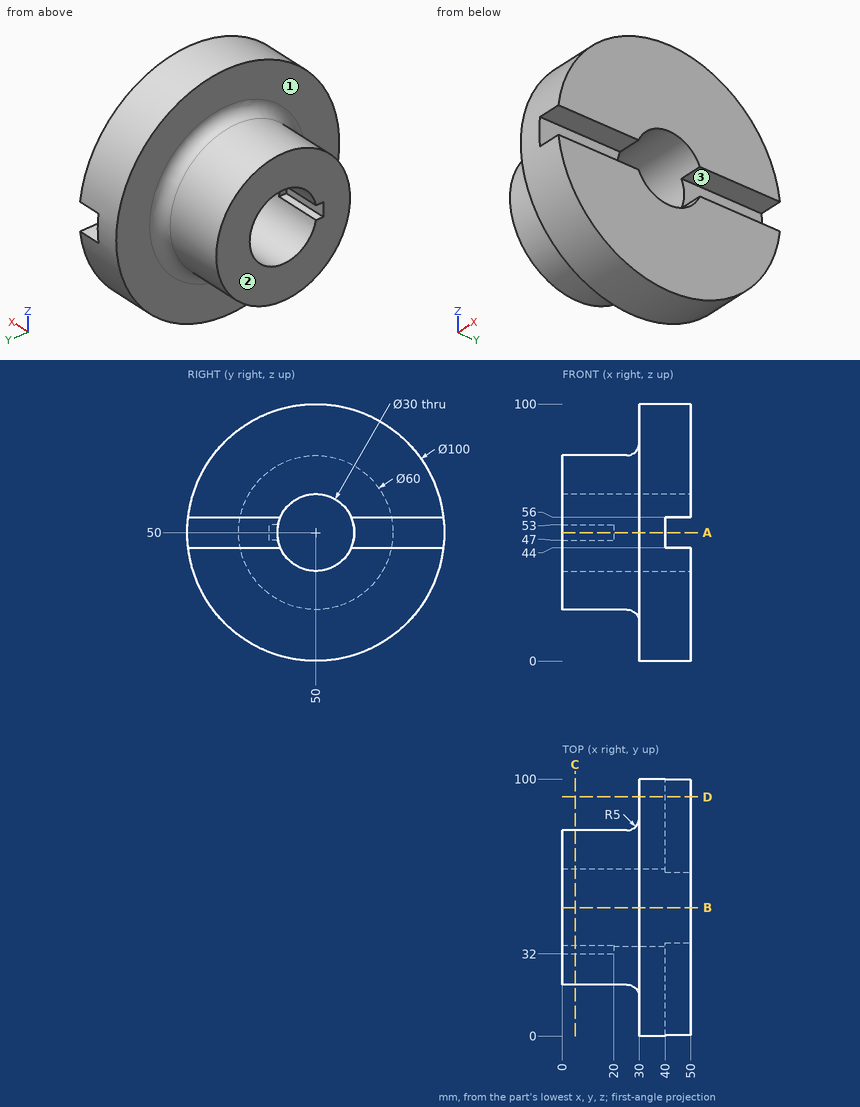
Geometry: see drawing. Coordinates: mm, zero at the bounding-box minimum. A direction names the side the tool comes from. Round coordinates to 2 decimals unless told otherwise and drop trailing zeros. Loops run counter-clockwise (first coordinate to the right, second up) from the corner with the lowest first, then second, coordinate; pieces in that order, holes last. Notation, with made-up numbers: (20.25, -20.5) -> (29.25, -20.5) arc R30 cw to (29.25, 14.5) -> close; hole circle Ø4 at (37.25, 10.25). An arc over 180 degrees is marked (long way). Write each question's results on one line, items separated by ' | '.
1. First-contact query: P1, Ø1.7, axis at y = 34, z = 49, coming from the -X side; P2, Ø3, axis at x = 39.5, z = 39, coming from the -Y side; P3, Ø11, axis at x = 44.5, y = 25, coming from the -Z side. Flat tips, straight axial feed; report the tip coordinate or a pass-through.
Geometry results:
P1: x = 20 | P2: y = 0.91 | P3: z = 3.96
2. Set-up query: the marked faces 1, 2 and 3. Return all of +Z, -Z, +X, -X, +Y, -Y with unobstructed straight access to the full face (end or side cutting, diameter ignored); none if empty.
Geometry results:
face 1: -X | face 2: +Z, -Z, -X, +Y, -Y | face 3: +X, +Y, -Y
3. Section A-A (z = 50). Return loops of the section in (x, y), and give its area (3 significant figures).
Geometry results:
outline: (0, 20) -> (25, 20) arc R5 cw to (30, 15) -> (30, 0) -> (40, 0) -> (40, 35) -> (20, 35) -> (20, 32) -> (0, 32) -> close; (0, 65) -> (40, 65) -> (40, 100) -> (30, 100) -> (30, 85) arc R5 cw to (25, 80) -> (0, 80) -> close | area: 1,550 mm2
4. Section C-C (x = 5). Return loops of the section in (y, z), and give its area (3 significant figures).
Geometry results:
outline: circle Ø60 at (50, 50); hole (32, 47) -> (35.3, 47) arc R15 ccw (long way) to (35.3, 53) -> (32, 53) -> close | area: 2,100 mm2
5. Ray query, line 1 (Z direction, x = 39, y = 50); line 2 (Z direction, x = 10, y = 50); line 3 (X direction, y = 45, z = 95). Return the intervals inside material, ascending. Write a range as from..to.
Geometry results:
line 1: 0..35, 65..100 | line 2: 20..35, 65..80 | line 3: 30..50
6. Section B-B (y = 50). Return loops of the section in (x, z).
Geometry results:
outline: (0, 20) -> (25, 20) arc R5 cw to (30, 15) -> (30, 0) -> (50, 0) -> (50, 35) -> (0, 35) -> close; (0, 65) -> (50, 65) -> (50, 100) -> (30, 100) -> (30, 85) arc R5 cw to (25, 80) -> (0, 80) -> close
7. Section D-D (y = 93). Return loops of the section in (x, z), and give its area (3 significant figures).
Geometry results:
outline: (30, 24.49) -> (50, 24.49) -> (50, 44) -> (40, 44) -> (40, 56) -> (50, 56) -> (50, 75.51) -> (30, 75.51) -> close | area: 901 mm2
